Job drawing, mm, ordinate dimensions from the low corner. One solid piece. A direction names the side the tool comes from. Round coordinates to 2 decimals unless told otherwise and drop trailing zeros. Order: outer loops, then holes, each group sorted by start corner. A loop starts at its lowest first (then second) coordinate and runs counter-clockwise, first axis right, second up. Notation, with made-up numbers: (-28.5, 40.25) -> (5.5, 40.25) arc R6 ccw to (5.5, 47.25) -> close; hole circle Ø7 at (87.5, 71.5). An arc over 180 degrees is marked (long way). Write item = value, one per line.
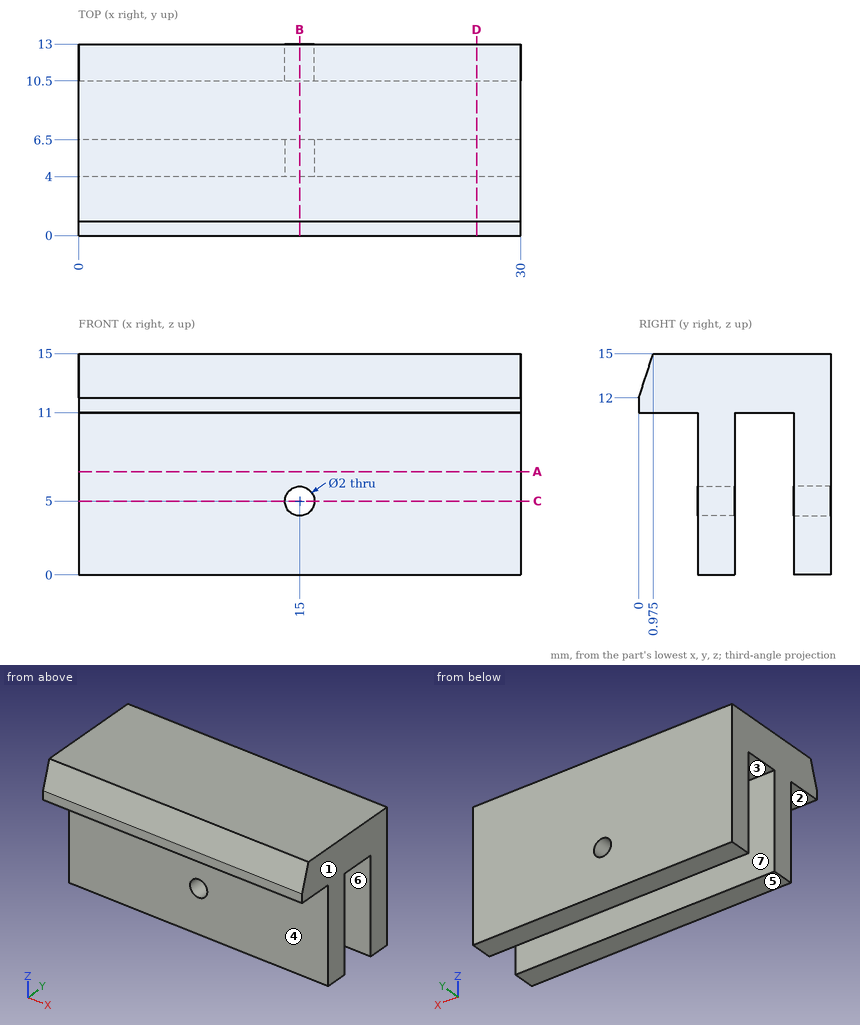
Q1. Cut at A-A, the plane z = 7. List the corners of the cut face in (x, y).
Check values:
outline = (0, 4) -> (30, 4) -> (30, 6.5) -> (0, 6.5) -> close; (0, 10.5) -> (30, 10.5) -> (30, 13) -> (0, 13) -> close
Q2. Cut at B-B, the plane x = 15. List the corners of the cut face in (y, z) (1 decimal).
Check values:
outline = (0, 11) -> (4, 11) -> (4, 6) -> (6.5, 6) -> (6.5, 11) -> (10.5, 11) -> (10.5, 6) -> (13, 6) -> (13, 15) -> (1, 15) -> (0, 12) -> close; (4, 0) -> (6.5, 0) -> (6.5, 4) -> (4, 4) -> close; (10.5, 0) -> (13, 0) -> (13, 4) -> (10.5, 4) -> close
Q3. Cut at D-D, the plane x = 27. List the corners of the cut face in (y, z) (1 decimal), and give its area (3 significant figures).
Check values:
outline = (0, 11) -> (4, 11) -> (4, 0) -> (6.5, 0) -> (6.5, 11) -> (10.5, 11) -> (10.5, 0) -> (13, 0) -> (13, 15) -> (1, 15) -> (0, 12) -> close
area = 106 mm²
Q4. Probe probe 1 along Y at (x, z) = (5.5, 7.5); probe 2 along X at (y, z) = (11.55, 5); probe 3 along Z at (x, y) = (20.75, 10). List the from-to ranges inside material, lowest first.
Check values:
probe_1 = 4 to 6.5, 10.5 to 13
probe_2 = 0 to 14, 16 to 30
probe_3 = 11 to 15
Q5. Flat gauge pins, fed straight in: pin 1 (5.5 mm diameter, centred on x = 19, z = 5, fed in from -Y); pin 2 (1.6 mm diameter, centred on x = 15, z = 5, fed in from +Y); pin 3 (1.5 mm diameter, centred on x = 22, y = 2, fed in from -Z). Where does each tip first touch, or does it go through?
Check values:
pin_1 = 4
pin_2 = through
pin_3 = 11
Q6. Cut at C-C, the plane z = 5. List the corners of the cut face in (x, y), and give its area (3 significant figures).
Check values:
outline = (0, 4) -> (14, 4) -> (14, 6.5) -> (0, 6.5) -> close; (0, 10.5) -> (14, 10.5) -> (14, 13) -> (0, 13) -> close; (16, 4) -> (30, 4) -> (30, 6.5) -> (16, 6.5) -> close; (16, 10.5) -> (30, 10.5) -> (30, 13) -> (16, 13) -> close
area = 140 mm²
Q7. Which spindle directions (+Z, -Z, +X, -X, +Y, -Y) get a long thin tool onto all of the face, cutting with end or side? Do the marked faces 1, 2 and 3. Say none if no direction does.
Check values:
face_1 = +Z, -Z, +X, +Y, -Y
face_2 = -Z, +X, -X, -Y
face_3 = -Z, +X, -X
Q8. Mould opens along Y. For the marked faces 4, 5, 6 and 7 say: released by +Y, released by -Y, zero draft, split by the parting line, or undercut.
Check values:
face_4 = released by -Y
face_5 = zero draft
face_6 = undercut
face_7 = undercut
